```python
from build123d import *

# Parameters (mm, degrees)
BOSS_EXTRUDE1_DEPTH      = 2.54
SKETCHED_START           = -165.1
SKETCHED_BEND1_OUTLINE_W = 228.6
SKETCHED_BEND1_OUTLINE_H = 2.54
SKETCHED_BEND1_DEPTH     = 125.300208363
SKETCHED_START_2         = -40.351159597
SKETCHED_BEND1_2_DEPTH   = 4.05656796
SKETCHED_START_3         = -114.3
SKETCHED_BEND1_3_DEPTH   = 228.6
SKETCHED_BEND1_4_DEPTH   = 228.6
SKETCH8_R                = 2.54
SKETCH8_R_2              = 3.175
SKETCH8_R_3              = 2.159
CUT_EXTRUDE2_DEPTH       = 2.54
SKETCH29_R               = 4.7625
CUT_EXTRUDE3_DEPTH       = 2.54


with BuildPart() as part:
    # Sketch2 → Boss-Extrude1 (new body)
    with BuildSketch(Plane.XY):
        with BuildLine():
            Line((109.22, -165.1), (-109.22, -165.1))
            ThreePointArc((-109.22, -165.1), (-112.812102448, -163.612102448), (-114.3, -160.02))
            Line((-114.3, -160.02), (-114.3, 160.02))
            ThreePointArc((-114.3, 160.02), (-112.812102448, 163.612102448), (-109.22, 165.1))
            Line((-109.22, 165.1), (109.22, 165.1))
            ThreePointArc((109.22, 165.1), (112.812102448, 163.612102448), (114.3, 160.02))
            Line((114.3, 160.02), (114.3, -160.02))
            ThreePointArc((114.3, -160.02), (112.812102448, -163.612102448), (109.22, -165.1))
        make_face()
    extrude(amount=BOSS_EXTRUDE1_DEPTH)

    # Sketched Bend1: read off the stored shape, not the designer's step
    # Sketched Bend1 outline → Sketched Bend1 (cut)
    with BuildSketch(Plane(origin=(0, 0, 0), x_dir=(1, 0, 0), z_dir=(0, 1, 0)).offset(SKETCHED_START)):
        with Locations((0, -1.27)):
            Rectangle(SKETCHED_BEND1_OUTLINE_W, SKETCHED_BEND1_OUTLINE_H)
    extrude(amount=SKETCHED_BEND1_DEPTH, mode=Mode.SUBTRACT)

    # Sketched Bend1 2 outline → Sketched Bend1 2 (add)
    with BuildSketch(Plane(origin=(0, 0, 0), x_dir=(1, 0, 0), z_dir=(0, 1, 0)).offset(SKETCHED_START_2)):
        with BuildLine():
            Line((114.3, -124.171159597), (114.3, -2.54))
            Line((114.3, -2.54), (-114.3, -2.54))
            Line((-114.3, -2.54), (-114.3, -124.171159597))
            ThreePointArc((-114.3, -124.171159597), (-112.812102448, -127.763262045), (-109.22, -129.251159597))
            Line((-109.22, -129.251159597), (109.22, -129.251159597))
            ThreePointArc((109.22, -129.251159597), (112.812102448, -127.763262045), (114.3, -124.171159597))
        make_face()
    extrude(amount=SKETCHED_BEND1_2_DEPTH)

    # Sketched Bend1 3 outline → Sketched Bend1 3 (cut)
    with BuildSketch(Plane.YZ.offset(SKETCHED_START_3)):
        with BuildLine():
            Line((-36.294591637, 129.251159597), (-37.811159597, 129.251159597))
            Line((-37.811159597, 129.251159597), (-37.811159597, 5.842))
            ThreePointArc((-37.811159597, 5.842), (-37.407322859, 4.259642992), (-36.294591637, 3.064332557))
            Line((-36.294591637, 3.064332557), (-36.294591637, 129.251159597))
        make_face()
        with BuildLine():
            ThreePointArc((-34.509159597, 0), (-38.640077413, 1.711082184), (-40.351159597, 5.842))
            Line((-40.351159597, 5.842), (-40.351159597, 2.54))
            Line((-40.351159597, 2.54), (-39.799791637, 2.54))
            Line((-39.799791637, 2.54), (-39.799791637, 0))
            Line((-39.799791637, 0), (-34.509159597, 0))
        make_face()
    extrude(amount=SKETCHED_BEND1_3_DEPTH, mode=Mode.SUBTRACT)

    # Sketched Bend1 4 outline → Sketched Bend1 4 (add)
    with BuildSketch(Plane.YZ.offset(SKETCHED_START_3)):
        with BuildLine():
            ThreePointArc((-34.509159597, 2.54), (-35.439575122, 2.673793733), (-36.294591637, 3.064332557))
            Line((-36.294591637, 3.064332557), (-36.294591637, 2.54))
            Line((-36.294591637, 2.54), (-34.509159597, 2.54))
        make_face()
    extrude(amount=SKETCHED_BEND1_4_DEPTH)

    # Sketch8 → Cut-Extrude2 (cut)
    with BuildSketch(Plane(origin=(0, -37.811159597, 0), x_dir=(1, 0, 0), z_dir=(0, 1, 0))):
        with Locations(Location((-104.14, -25.111159597, 0), (0, 0, 270))):
            Circle(SKETCH8_R)
        with Locations(Location((0.508, -25.111159597, 0), (0, 0, 270))):
            Circle(SKETCH8_R)
        with Locations(Location((-104.14, -101.565159597, 0), (0, 0, 270))):
            Circle(SKETCH8_R)
        with Locations(Location((-27.94, -101.565159597, 0), (0, 0, 270))):
            Circle(SKETCH8_R)
        with Locations(Location((-66.04, -63.211159597, 0), (0, 0, 270))):
            Circle(SKETCH8_R_2)
        with Locations(Location((68.326, -48.225159597, 0), (0, 0, 270))):
            Circle(SKETCH8_R_3)
        with Locations(Location((98.044, -48.225159597, 0), (0, 0, 270))):
            Circle(SKETCH8_R_3)
        with Locations(Location((98.044, -79.721159597, 0), (0, 0, 270))):
            Circle(SKETCH8_R_3)
        with Locations(Location((68.326, -79.721159597, 0), (0, 0, 270))):
            Circle(SKETCH8_R_3)
    extrude(amount=-CUT_EXTRUDE2_DEPTH, mode=Mode.SUBTRACT)

    # Sketch29 → Cut-Extrude3 (cut)
    with BuildSketch(Plane.XY.offset(2.54)):
        with Locations((-82.55, 146.05)):
            Circle(SKETCH29_R)
        with Locations((82.55, 146.05)):
            Circle(SKETCH29_R)
        with Locations((38.1, 0)):
            Circle(SKETCH29_R)
    extrude(amount=-CUT_EXTRUDE3_DEPTH, mode=Mode.SUBTRACT)


solid = part.part
```
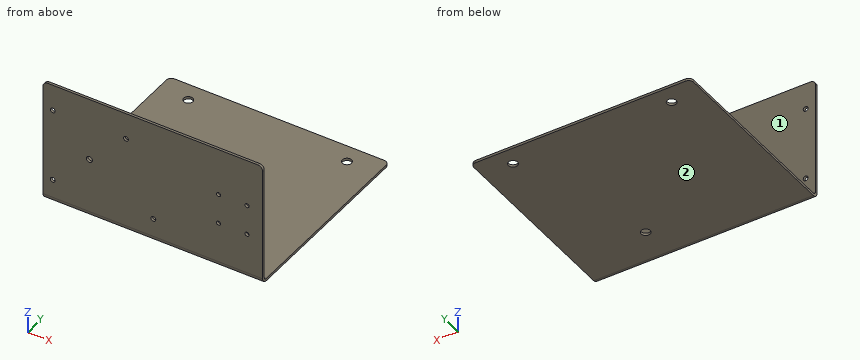
Input: part model. Units: mm. Frame: model coordinates. Face numbers are marked on the shaded views. A direction names the side the tool comes from. Coordinates: 2 decimals unless noted, no trailing zeros. Write each loop counter-clockwise with the first axis right and the second up, starting at its lowest first coordinate (ties: lowest second). Pieces come first, ordered by that corner, then holes. Notation, with made-up numbers: (-36, 63.5) - (-31, 63.5) arc R9 cw to (-31, 70.5) - close; hole circle Ø1 at (43.25, -20.5). An arc over 180 degrees is marked (long way). Put each result on its own line as item: value. Start each with the question number.
1) Cut plane C-C (x = -82.55). Return the cut outline in (y, z), plus the area to 3 significant figures.
2) Cut plane B-B (y = 146.05). Return the cut outline in (x, z).
3) Cut plane A-A (y = 0). Return the cut outline in (x, z).
4) Ray query, L1, parallel to Y at x = 22.5, z = 71.5; L2, parallel to Z at x = -64, y = -28.5; L3, parallel to Z at x = -27, y = -39. Return the intervals inside material, ascending.
5) Reachability of the marked faces 1 and 2 from +Z, -Z, +X, -X, +Y, -Y: full face, straight path, thin tool, end or side. Return the list, or none.
6) Cut plane D-D (x = 11.5). Return the cut outline in (y, z).
7) Contact query for flat-ended pins moving along their axis: pin 1 (10 mm diameter, centred on x = 18.5, z = 57, fed in from +Y); pin 2 (7.5 mm diameter, centred on x = 82.55, y = 146.05, fed in from +Z); pin 3 (12.5 mm diameter, centred on x = 38.1, y = 0, fed in from +Z). Output: stop coordinate, or through.
Resolved:
1. outline: (-40.35, 5.84) arc R5.84 ccw to (-34.51, 0) - (141.29, 0) - (141.29, 2.54) - (-34.51, 2.54) arc R3.3 cw to (-37.81, 5.84) - (-37.81, 129.25) - (-40.35, 129.25) - close; (150.81, 0) - (165.1, 0) - (165.1, 2.54) - (150.81, 2.54) - close
1. area: 815 mm2
2. outline: (-114.3, 0) - (-87.31, 0) - (-87.31, 2.54) - (-114.3, 2.54) - close; (-77.79, 0) - (77.79, 0) - (77.79, 2.54) - (-77.79, 2.54) - close; (87.31, 0) - (114.3, 0) - (114.3, 2.54) - (87.31, 2.54) - close
3. outline: (-114.3, 0) - (33.34, 0) - (33.34, 2.54) - (-114.3, 2.54) - close; (42.86, 0) - (114.3, 0) - (114.3, 2.54) - (42.86, 2.54) - close
4. L1: y = -40.35 to -37.81
4. L2: z = 0 to 2.54
4. L3: z = 2.11 to 99.21, 103.92 to 129.25
5. face 1: +Z, +X, -X, +Y
5. face 2: -Z, +X, -X, +Y, -Y
6. outline: (-40.35, 5.84) arc R5.84 ccw to (-34.51, 0) - (165.1, 0) - (165.1, 2.54) - (-34.51, 2.54) arc R3.3 cw to (-37.81, 5.84) - (-37.81, 129.25) - (-40.35, 129.25) - close
7. pin 1: stops at y = -37.81
7. pin 2: passes through
7. pin 3: stops at z = 2.54
